from build123d import *

# Parameters (mm, degrees)
F1_DEPTH = 76.2
F3_D     = 12.7
F5_DEPTH = 15.494
F6_W     = 17.5469946116
F6_H     = 6.365576759
F7_DEPTH = 76.2
F9_D     = 12.7


with BuildPart() as f1:
    # F0 (on Front) → F1 (new body)
    with BuildSketch(Plane.XZ):
        Polygon((-12.2837694362, 17.4164939672), (-57.7873364091, 17.4164939672), (-57.7873364091, -13.6970570311), (-12.2837694362, -13.6970570311), (-12.2837694362, -22.2532823682), (14.5516674966, -22.2532823682), (14.5516674966, 3.3165175266), align=None)
        Polygon((33.6087159812, -6.6965087317), (14.5516674966, 3.3165175266), (14.5516674966, -22.2532823682), (33.6087159812, -22.2532823682), align=None)
    extrude(amount=F1_DEPTH)

    # F3 (through all)
    with Locations(Plane.XY.offset(17.4164939672)):
        with Locations((-42.3829220235, -14.8011986166), (-28.5008102655, -57.2022236884)):
            Hole(F3_D / 2)

    # F4 (on face) → F5 (cut)
    with BuildSketch(Plane.XZ.offset(76.2)):
        Polygon((33.6087159812, -6.6965087317), (17.0117028464, 2.023956479), (17.0117028464, -22.2532823682), (33.6087159812, -22.2532823682), align=None)
    extrude(amount=-F5_DEPTH, mode=Mode.SUBTRACT)

    # F6 (on face) → F7 (cut)
    with BuildSketch(Plane.YZ.offset(33.6087159812)):
        with Locations((-31.9253103808, -19.0704939887)):
            Rectangle(F6_W, F6_H)
    extrude(amount=-F7_DEPTH, mode=Mode.SUBTRACT)

    # F9 (through all)
    with Locations(Plane(origin=(4.5137471869, 0, 8.5906794578), x_dir=(0.8852434605, 0, -0.4651279563), z_dir=(0.4651279563, 0, 0.8852434605))):
        with Locations((0, -33.5651822388)):
            Hole(F9_D / 2)


solid = f1.part
CAD build for the part. Positions are in the model's coordinates, mm. A direction names the side the tool comes from. Round coordinates to 2 decimals unless told otherwise and drop trailing zeros. Write each loop counter-clockwise with the first axis right and the second up, starting at its lowest first coordinate (ties: lowest second). Pieces come first, ordered by that corner, then holes. Notation, with made-up numbers: M 44.5,55 L 53.5,55 A18 cw 53.5,65 Z; hole C 86,-25.75 d9. An arc over 180 degrees is marked long. Use a Markdown table: item, result. Add a question column.
1. Slice it at B-B on y = -16. Give the cut face in (x, z).
2. Slice it at C-C on x = -33. Give the cut face in (y, z).
3. 3-axis set-ups, long thin cutter, end or side, ignore diameter. For faces 1 (the face through (-35, -38, 17.416)), 2 (the face through (11, -23.152, -19)), 3 (the face through (25, -60.706, -13)), 4 (the face through (-12.284, -57, -18)): which of +Z, -Z, +X, -X, +Y, -Y reach the whole face in a straight line?
4. Pull direction X, two halves, no side cores. Call faces 5 (the face through (-35, -38, -13.697)), 6 (the face through (17.012, -69, -10)), 7 (the face through (-7.63, -36, -1.91)): released by +X, released by -X, zero draft, split by the parting line, or undercut.
5. Flat gauge pins, fed straight in: P1, Ø10, axis at x = -28.5, y = -57.2, coming from the -Z side; P2, Ø8, axis at x = -29.5, y = -63.5, coming from the -Z side; P3, Ø14, axis at x = 6, y = -31, coming from the -Z side; P4, Ø8.5, axis at x = 29, z = -5.5, coming from the -Y side. Where does each tip first touch, or does it go through?
6. Drill centre lines: probe 1 along Y at (x, z) = (18, -5); probe 2 along Y at (x, z) = (3, -17.5); probe 3 along X at (y, z) = (-10.5, 9). Where is each one in solid material? Low to high.
7. Slice it at D-D on y = -36.5. Give the cut face in (x, z).
8. Slice it at A-A on z = -18. Give the cut face in (x, y), then the cut area to 3 significant figures.
Reply:
| question | item | result |
|---|---|---|
| 1 | outline | M -57.79,-13.7 L -48.62,-13.7 L -48.62,17.42 L -57.79,17.42 Z; M -36.15,-13.7 L -12.28,-13.7 L -12.28,-22.25 L 33.61,-22.25 L 33.61,-6.7 L -12.28,17.42 L -36.15,17.42 Z |
| 2 | outline | M -76.2,-13.7 L -61.68,-13.7 L -61.68,17.42 L -76.2,17.42 Z; M -52.72,-13.7 L 0,-13.7 L 0,17.42 L -52.72,17.42 Z |
| 3 | face 1 | +Z, +X, -X, +Y, -Y |
| 3 | face 2 | -Z, +X, -X |
| 3 | face 3 | +Z, -Z, +X, -Y |
| 3 | face 4 | -Z, -X, +Y, -Y |
| 4 | face 5 | zero draft |
| 4 | face 6 | released by +X |
| 4 | face 7 | undercut |
| 5 | P1 | passes through |
| 5 | P2 | stops at z = -13.7 |
| 5 | P3 | stops at z = -15.89 |
| 5 | P4 | stops at y = -60.71 |
| 6 | probe 1 | y = -60.71 to 0 |
| 6 | probe 2 | y = -76.2 to -40.7, -23.15 to 0 |
| 6 | probe 3 | x = -57.79 to -47.05, -37.71 to 3.73 |
| 7 | outline | M -57.79,-13.7 L -13.56,-13.7 L -0.47,11.21 L -12.28,17.42 L -57.79,17.42 Z; M -1.99,-15.89 L 33.61,-15.89 L 33.61,-6.7 L 9.5,5.97 Z |
| 8 | outline | M -12.28,-76.2 L 17.01,-76.2 L 17.01,-60.71 L 33.61,-60.71 L 33.61,-40.7 L -12.28,-40.7 Z; M -12.28,-23.15 L 33.61,-23.15 L 33.61,0 L -12.28,0 Z |
| 8 | area | 2,430 mm^2 |
